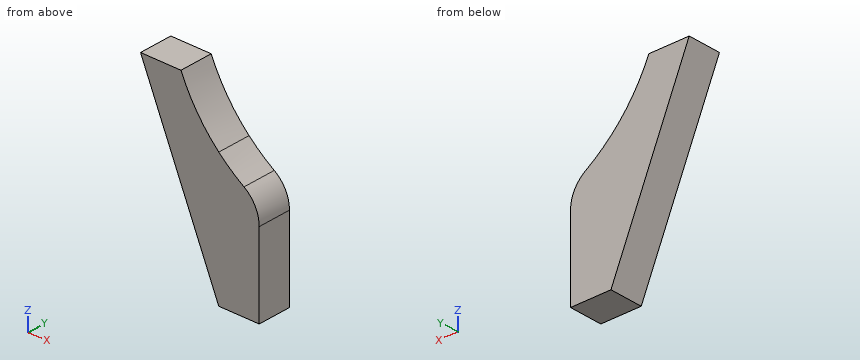
```python
from build123d import *

# Parameters (mm, degrees)
EXTRUDE_2_DEPTH     = 5
SKETCH_4_R          = 1.65
CUT_EXTRUDE_1_DEPTH = 5
EXTRUDE_3_DEPTH     = 5
CUT_EXTRUDE_START   = -4.5
SKETCH_7_R          = 3
CUT_EXTRUDE_2_DEPTH = 3
CUT_EXTRUDE_3_DEPTH = 7.5
EXTRUDE_4_DEPTH     = 5
FILLET_1_R          = 5
FILLET_2_R          = 5
SKETCH_10_R         = 1.65
CUT_EXTRUDE_4_DEPTH = 5


with BuildPart() as part:
    # 草图3 → 凸台-拉伸2 (new body)
    with BuildSketch(Plane(origin=(0, 0, 0), x_dir=(1, 0, 0), z_dir=(0, 1, 0))):
        with BuildLine():
            Line((-3, -3.354101966), (-3, -7.416198487))
            Line((-3, -7.416198487), (-3, -43.854101966))
            Line((-3, -43.854101966), (3, -43.854101966))
            Line((3, -43.854101966), (3, -10.583005244))
            Line((3, -10.583005244), (3, -7.416198487))
            Line((3, -7.416198487), (3, -3.354101966))
            ThreePointArc((3, -3.354101966), (0, 4.5), (-3, -3.354101966))
        make_face()
    extrude(amount=EXTRUDE_2_DEPTH)

    # 草图4 → 切除-拉伸1 (cut)
    with BuildSketch(Plane(origin=(0, 5, 0), x_dir=(1, 0, 0), z_dir=(0, 1, 0))):
        with Locations(Location((0, 0, 0), (0, 0, 270))):
            Circle(SKETCH_4_R)
    extrude(amount=-CUT_EXTRUDE_1_DEPTH, mode=Mode.SUBTRACT)

    # 草图6 → 凸台-拉伸3 (add)
    with BuildSketch(Plane(origin=(0, 5, 0), x_dir=(1, 0, 0), z_dir=(0, 1, 0))):
        with BuildLine():
            Line((3, -33.74604712), (-3, -33.74604712))
            ThreePointArc((-3, -33.74604712), (-16.46902092, -57.986607816), (0.722500961, -79.745993902))
            Line((0.722500961, -79.745993902), (1.949520222, -77.620734201))
            ThreePointArc((1.949520222, -77.620734201), (-10.543317179, -55.371702353), (3, -33.74604712))
        make_face()
    extrude(amount=-EXTRUDE_3_DEPTH)

    # 草图7 → 切除-拉伸2 (cut)
    with BuildSketch(Plane(origin=(0, 5, 0), x_dir=(1, 0, 0), z_dir=(0, 1, 0)).offset(CUT_EXTRUDE_START)):
        with Locations(Location((0, 0, 0), (0, 0, 270))):
            Circle(SKETCH_7_R)
    extrude(amount=-CUT_EXTRUDE_2_DEPTH, mode=Mode.SUBTRACT)

    # 草图8 → 切除-拉伸3 (cut)
    with BuildSketch(Plane(origin=(0, 5, 0), x_dir=(1, 0, 0), z_dir=(0, 1, 0))):
        with BuildLine():
            Line((-3, -38.067187498), (-3, -43.854101966))
            Line((-3, -43.854101966), (3, -43.854101966))
            Line((3, -43.854101966), (3, -33.74604712))
            ThreePointArc((3, -33.74604712), (-0.160637142, -35.683569047), (-3, -38.067187498))
        make_face()
    extrude(amount=-CUT_EXTRUDE_3_DEPTH, mode=Mode.SUBTRACT)

    # 草图9 → 凸台-拉伸4 (add)
    with BuildSketch(Plane(origin=(0, 5, 0), x_dir=(1, 0, 0), z_dir=(0, 1, 0))):
        with BuildLine():
            Line((-3, -18.550074543), (-14.614967684, -46.324924269))
            ThreePointArc((-14.614967684, -46.324924269), (-9.917875534, -39.010182445), (-3, -33.74604712))
            Line((-3, -33.74604712), (-3, -18.550074543))
        make_face()
    extrude(amount=-EXTRUDE_4_DEPTH)

    # 圆角1
    fillet_1_edges = [part.edges().sort_by_distance(p)[0] for p in [
        (3, 2.5, 33.74604712),
    ]]
    fillet(fillet_1_edges, radius=FILLET_1_R)

    # 圆角2
    # the kernel refuses this fillet: 5 mm, written as the material it takes off along each edge
    with BuildSketch(Plane(origin=(1.949520222, 14.371610933, 77.620734201), x_dir=(-0.8261015944022844, 0, -0.5635212114250925), z_dir=(0, -1, 0))) as fillet_2_piece_1:
        with BuildLine():
            CenterArc((4.123508811, -4.985927863), FILLET_2_R, 94.299664485, 55.185648669)
            Line((-0.183986354, -2.447131808), (-0.270136257, -2.396355887))
            ThreePointArc((-0.270136257, -2.396355887), (-0.191711734, -1.216068615), (-0.099718557, 0.007497289))
            Line((-0.099718557, 0.007497289), (0.007497289, 0.099718557))
            ThreePointArc((0.007497289, 0.099718557), (1.874322187, 0.029639314), (3.741147084, 0.099718557))
            Line((3.741147084, 0.099718557), (3.748644373, 0))
        make_face()
    extrude(amount=23.743221866, mode=Mode.SUBTRACT)

    # 草图10 → 切除-拉伸4 (cut)
    # profile 1 of 2: a face of its own
    with BuildSketch(Plane(origin=(0, 5, 0), x_dir=(1, 0, 0), z_dir=(0, 1, 0))):
        with BuildLine():
            Line((-3, -3.354101966), (-3, -18.550074543))
            Line((-3, -18.550074543), (3, -18.550074543))
            Line((3, -18.550074543), (3, -3.354101966))
            ThreePointArc((3, -3.354101966), (0, 4.5), (-3, -3.354101966))
        make_face()
        Circle(SKETCH_10_R, mode=Mode.SUBTRACT)
    # profile 2 of 2: a face of its own
    with BuildSketch(Plane(origin=(0, 5, 0), x_dir=(1, 0, 0), z_dir=(0, 1, 0))):
        with BuildLine():
            Line((-8.614967684, -46.324924269), (-14.614967684, -46.324924269))
            ThreePointArc((-14.614967684, -46.324924269), (-14.272081884, -66.397409294), (0.722500961, -79.745993902))
            ThreePointArc((0.722500961, -79.745993902), (0.307928877, -77.397579493), (-1.147240872, -75.508293582))
            ThreePointArc((-1.147240872, -75.508293582), (-9.770106213, -62.167654699), (-8.614967684, -46.324924269))
        make_face()
    extrude(amount=-CUT_EXTRUDE_4_DEPTH, mode=Mode.SUBTRACT)


solid = part.part
```
Geometry check sheet. Reference: the model listing, model coordinates, mm. Give positions to 0.01 mm unless a question says otherwise; leave off trailing zeros. Loops run counter-clockwise (first coordinate to the right, second up) from the corner with the lowest first, then second, coordinate; pieces in that order, holes last. Notation, with made-up numbers: M -1.5,-29 L 30.5,-29 A20 ccw 30.5,-4 Z; hole C 23,-10.5 d6. An arc over 180 degrees is marked long. Answer as CSV lines item,"result".
Item 1: Cross-section at C-C on x = -0.5. Record the cut outline in (y, z).
Values:
outline,"M 0,18.55 L 5,18.55 L 5,35.93 L 0,35.93 Z"
Item 2: Cross-section at B-B on z = 40.25. Record the cut outline in (x, y), and give its area (3 significant figures).
Values:
outline,"M -12.07,0 L -4.99,0 L -4.99,5 L -12.07,5 Z"
area,"35.4 mm²"
Item 3: Material ranges on line 1 (X direction, y = 2, z = 36.25); line 2 (Z direction, x = -2.5, y = 1.55); line 3 (Z direction, x = -12.5, y = 1), recorded low to high.
Values:
line 1,"x = -10.4 to -0.92"
line 2,"z = 18.55 to 37.59"
line 3,"z = 41.27 to 46.32"
Item 4: Cross-section at A-A on y = 4.4. Record the cut outline in (x, z).
Values:
outline,"M -14.61,46.32 L -3,18.55 L 3,18.55 L 3,30.88 A5 ccw 0.74,35.06 A25 cw -8.61,46.32 Z"
Item 5: Depth check by flat-ended pin: P1, Ø3, axis at x = -1, y = 3, coming from the +Z side; P2, Ø3, axis at y = 1, z = 41, coming from the -X side; P3, Ø1.5, axis at y = 2, z = 22.5, coming from the -X side; P4, Ø1.5, axis at x = -9.5, z = 38.5, coming from the -Y side. Enter the tip coordinate at first touch or a pass-through.
Values:
P1,"stops at z = 37.59"
P2,"stops at x = -13.02"
P3,"stops at x = -4.97"
P4,"stops at y = 0"
